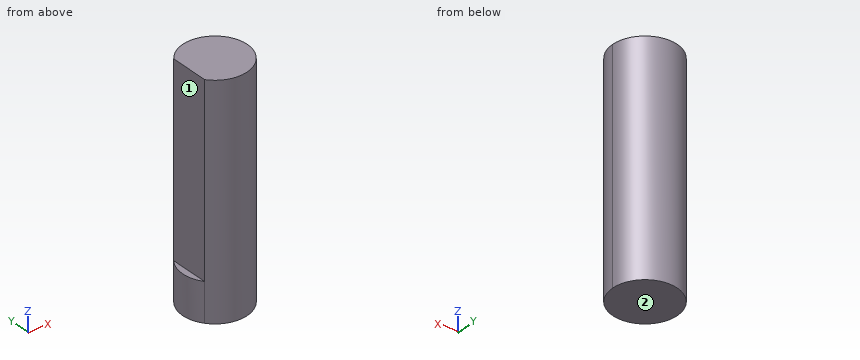
```python
from build123d import *

# Parameters (mm, degrees)
F1_DEPTH = 17.5
F2_DEPTH = 3


with BuildPart() as f1:
    # F0 (on Top) → F1 (new body)
    with BuildSketch(Plane.XY):
        with BuildLine():
            ThreePointArc((-2, -1.5), (0.790569, -2.371708), (2.5, 0))
            ThreePointArc((2.5, 0), (0.790569, 2.371708), (-2, 1.5))
            Line((-2, 1.5), (-2, -1.5))
        make_face()
    extrude(amount=F1_DEPTH)

    # F0 (on Top) → F2 (join)
    with BuildSketch(Plane.XY):
        with BuildLine():
            Line((-2, -1.5), (-2, 1.5))
            ThreePointArc((-2, 1.5), (-2.5, 0), (-2, -1.5))
        make_face()
    extrude(amount=F2_DEPTH)


solid = f1.part
```
Check sheet for the modelled part. Datum: model origin and axes. Units: mm. Face numbers are marked on the shaded views. A direction names the side the tool comes from. Coordinates: 2 decimals unless noted, no trailing zeros. Write each loop counter-clockwise with the first axis right and the second up, starting at its lowest first coordinate (ties: lowest second). Pieces come first, ordered by that corner, then holes. Notation, with made-up numbers: (53.25, 41.25) -> (82.25, 41.25) arc R12 ccw to (82.25, 45.25) -> close; hole circle Ø2 at (-22, -25.5). An arc over 180 degrees is marked (long way). Use a Markdown table: item, result.
1. Sectioned sample at D-D (y = 1.75). Enter the section's corners in (x, z), plus the area to 3 significant figures.
Reported:
| item | result |
|---|---|
| outline | (-1.79, 0) -> (1.79, 0) -> (1.79, 17.5) -> (-1.79, 17.5) -> close |
| area | 62.5 mm2 |
2. Tool access check on the marked faces 1 and 2. Record the directions out of +Z, -Z, +X, -X, +Y, -Y that give a thin tool (end or side, any length) a straight path to the whole face; none if there is none.
Reported:
| item | result |
|---|---|
| face 1 | +Z, -X, +Y, -Y |
| face 2 | -Z, +X, -X, +Y, -Y |
3. Sectioned sample at B-B (x = 1.5). Enter the section's corners in (y, z).
Reported:
| item | result |
|---|---|
| outline | (-2, 0) -> (2, 0) -> (2, 17.5) -> (-2, 17.5) -> close |
4. Sectioned sample at A-A (y = 0.7). Enter the section's corners in (x, z).
Reported:
| item | result |
|---|---|
| outline | (-2.4, 0) -> (2.4, 0) -> (2.4, 17.5) -> (-2, 17.5) -> (-2, 3) -> (-2.4, 3) -> close |
5. Sectioned sample at C-C (z = 7.25). Enter the section's corners in (x, y).
Reported:
| item | result |
|---|---|
| outline | (-2, -1.5) arc R2.5 ccw to (2.5, 0) arc R2.5 ccw to (-2, 1.5) -> close |
6. Scan lines: line 1 along Y through (x, z) = (2, 16.5); line 2 along X through (y, z) = (-0.05, 9.5); line 3 along Y through (x, z) = (-0.1, 3.75). Record each from-to range of solid material in increasing order.
Reported:
| item | result |
|---|---|
| line 1 | y = -1.5 to 1.5 |
| line 2 | x = -2 to 2.5 |
| line 3 | y = -2.5 to 2.5 |
7. Go/stop test with a flat-tipped pin: pin 1 Ø2.5 at (y, z) = (0.5, 7.5) entering from -X. Record where the tip stops, or that it passes through.
Reported:
| item | result |
|---|---|
| pin 1 | stops at x = -2 |
